Read the model definition and answer for the solid it produces. Units are mm, in the model's axes. A direction names the side the tool comes from. Coordinates: 2 decimals unless noted, no trailing zeros. Write each loop counter-clockwise with the first axis right and the second up, starting at its lowest first coordinate (ties: lowest second). Pieces come first, ordered by that corner, then holes.
(1) Which of the six approach directions +Z, -Z, +X, -X, +Y, -Y give full straight-line access (tool end or side, diameter ignored) to faces 4 (the flat face through (2, -37, 0)), 5 (the flat face through (9, -35, 50))?
(2) The part is cut by section A-A, the plane y = -33.5. Determine the outline of the cut face in (x, z).
(3) Given pin 1 (4 mm diameter, centred on x = -1, z = 34.5, fed in from +Y); pin 2 (0.7 mm diameter, centred on x = 0, z = 62.5, fed in from +Y), each flat-ended and moving along its own axis, determine where each tip first touches the part or whether it passes through.
(4) Determine the mould class of faces 1 (the flat face through (-7, -36, 50)), 2 (the flat face through (1, -35, 50)), 3 (the flat face through (2, -31.87, 50)) for opening direction X: pulls with the +X half, pulls with the -X half, needs draft (parallel to the pull), parting line crosses it, or undercut.
(5) Straight lines are drawn through the part: line 1 along X through (y, z) = (-33.5, 39); line 2 along X through (y, z) = (-37.75, 80); line 3 along Y through (x, z) = (-3, 63). For each, find the intervals that lie inside material, in ascending order.
```python
from build123d import *

# Parameters (mm, degrees)
ESBO_O1_W                = 3
ESBO_O1_H                = 6
RESSALTO_EXTRUS_O1_DEPTH = 102
ESBO_O1_6_W              = 2
ESBO_O1_6_H              = 6
RESSALTO_EXTRUS_O3_DEPTH = 102
RESSALTO_EXTRUS_O4_DEPTH = 102
FILETE3_R                = 0.6


with BuildPart() as part:
    # Esbo_o1 → Ressalto-extrus_o1 (new body)
    with BuildSketch(Plane.XY):
        with Locations((-2, -34.87037037)):
            Rectangle(ESBO_O1_W, ESBO_O1_H)
    extrude(amount=RESSALTO_EXTRUS_O1_DEPTH)

    # Esbo_o1_6 → Ressalto-extrus_o3 (add)
    with BuildSketch(Plane.XY):
        with Locations((-6, -34.87037037)):
            Rectangle(ESBO_O1_6_W, ESBO_O1_6_H)
        with BuildLine():
            Line((-5, -37.87037037), (-4.698132677, -37.87037037))
            ThreePointArc((-4.698132677, -37.87037037), (-4.911585108, -37.781955478), (-5, -37.568503047))
            Line((-5, -37.568503047), (-5, -37.87037037))
        make_face()
        with BuildLine():
            Line((-3.801867323, -37.87037037), (-3.5, -37.87037037))
            Line((-3.5, -37.87037037), (-3.5, -37.568503047))
            ThreePointArc((-3.5, -37.568503047), (-3.588414892, -37.781955478), (-3.801867323, -37.87037037))
        make_face()
        with BuildLine():
            Line((-0.5, -37.568503047), (-0.5, -37.87037037))
            Line((-0.5, -37.87037037), (-0.198132677, -37.87037037))
            ThreePointArc((-0.198132677, -37.87037037), (-0.411585108, -37.781955478), (-0.5, -37.568503047))
        make_face()
        with BuildLine():
            ThreePointArc((1, -37.568503047), (0.911585108, -37.781955478), (0.698132677, -37.87037037))
            Line((0.698132677, -37.87037037), (1, -37.87037037))
            Line((1, -37.87037037), (1, -37.568503047))
        make_face()
        with Locations((2, -34.87037037)):
            Rectangle(ESBO_O1_6_W, ESBO_O1_6_H)
        with BuildLine():
            Line((3, -37.568503047), (3, -37.87037037))
            Line((3, -37.87037037), (3.301867323, -37.87037037))
            ThreePointArc((3.301867323, -37.87037037), (3.088414892, -37.781955478), (3, -37.568503047))
        make_face()
        with BuildLine():
            ThreePointArc((4.5, -37.568503047), (4.411585108, -37.781955478), (4.198132677, -37.87037037))
            Line((4.198132677, -37.87037037), (4.5, -37.87037037))
            Line((4.5, -37.87037037), (4.5, -37.568503047))
        make_face()
        Polygon((4.5, -37.568503047), (4.5, -37.87037037), (6, -37.87037037), (6, -31.87037037), (4.5, -31.87037037), align=None)
        Polygon((6, -31.87037037), (6, -37.87037037), (7.5, -37.87037037), (7.5, -37.568503047), (7.5, -31.87037037), align=None)
        with BuildLine():
            Line((7.5, -37.87037037), (7.801867323, -37.87037037))
            ThreePointArc((7.801867323, -37.87037037), (7.588414892, -37.781955478), (7.5, -37.568503047))
            Line((7.5, -37.568503047), (7.5, -37.87037037))
        make_face()
        with BuildLine():
            Line((8.698132677, -37.87037037), (9, -37.87037037))
            Line((9, -37.87037037), (9, -37.568503047))
            ThreePointArc((9, -37.568503047), (8.911585108, -37.781955478), (8.698132677, -37.87037037))
        make_face()
        with Locations((10, -34.87037037)):
            Rectangle(ESBO_O1_6_W, ESBO_O1_6_H)
    extrude(amount=RESSALTO_EXTRUS_O3_DEPTH)

    # Esbo_o1_7 → Ressalto-extrus_o4 (add)
    with BuildSketch(Plane.XY):
        Polygon((-2, -37.87037037), (-3.5, -37.87037037), (-3.801867323, -37.87037037), (-4.698132677, -37.87037037), (-5, -37.87037037), (-7, -37.87037037), (-7, -39.87037037), (11, -39.87037037), (11, -37.87037037), (9, -37.87037037), (8.698132677, -37.87037037), (7.801867323, -37.87037037), (7.5, -37.87037037), (6, -37.87037037), (4.5, -37.87037037), (4.198132677, -37.87037037), (3.301867323, -37.87037037), (3, -37.87037037), (1, -37.87037037), (0.698132677, -37.87037037), (-0.198132677, -37.87037037), (-0.5, -37.87037037), align=None)
    extrude(amount=RESSALTO_EXTRUS_O4_DEPTH)

    # Filete3
    filete3_edges = [part.edges().sort_by_distance(p)[0] for p in [
        (7.5, -31.87037037, 51),
        (4.5, -31.87037037, 51),
        (-0.5, -31.87037037, 51),
        (-3.5, -31.87037037, 51),
    ]]
    fillet(filete3_edges, radius=FILETE3_R)


solid = part.part
```
Computed:
1. face 4: -Z, +X, -X, +Y, -Y
1. face 5: +Z, -Z, +Y
2. outline: (-7, 0) - (-5, 0) - (-5, 102) - (-7, 102) - close; (-3.5, 0) - (-0.5, 0) - (-0.5, 102) - (-3.5, 102) - close; (1, 0) - (3, 0) - (3, 102) - (1, 102) - close; (4.5, 0) - (7.5, 0) - (7.5, 102) - (4.5, 102) - close; (9, 0) - (11, 0) - (11, 102) - (9, 102) - close
3. pin 1: stops at y = -31.87
3. pin 2: stops at y = -37.83
4. face 1: pulls with the -X half
4. face 2: undercut
4. face 3: needs draft
5. line 1: x = -7 to -5, -3.5 to -0.5, 1 to 3, 4.5 to 7.5, 9 to 11
5. line 2: x = -7 to -4.94, -3.56 to -0.44, 0.94 to 3.06, 4.44 to 7.56, 8.94 to 11
5. line 3: y = -39.87 to -31.88
